```python
from build123d import *

# Parameters (mm, degrees)
SKETCH1_W           = 51
SKETCH1_H           = 36
BOSS_EXTRUDE1_DEPTH = 3
SKETCH2_W           = 45
SKETCH2_H           = 30
BOSS_EXTRUDE2_DEPTH = 10
FILLET1_R           = 1.8
FILLET2_R           = 2.2
CHAMFER1_SIZE       = 1
SKETCH3_R           = 15
CUT_EXTRUDE1_DEPTH  = 10
SKETCH4_R           = 1.25
CUT_EXTRUDE2_DEPTH  = 50
CHAMFER2_SIZE       = 1
SKETCH5_R           = 4.5
BOSS_EXTRUDE3_DEPTH = 7


with BuildPart() as part:
    # Sketch1 → Boss-Extrude1 (new body)
    with BuildSketch(Plane(origin=(0, 0, 0), x_dir=(1, 0, 0), z_dir=(0, 1, 0))):
        Rectangle(SKETCH1_W, SKETCH1_H)
    extrude(amount=BOSS_EXTRUDE1_DEPTH)

    # Sketch2 → Boss-Extrude2 (add)
    with BuildSketch(Plane(origin=(0, 3, 0), x_dir=(1, 0, 0), z_dir=(0, 1, 0))):
        Polygon((-22.5, 18), (-25.5, 18), (-25.5, 15), (-25.5, -15), (-25.5, -18), (-22.5, -18), (22.5, -18), (25.5, -18), (25.5, -15), (25.5, 15), (25.5, 18), (22.5, 18), align=None)
        Rectangle(SKETCH2_W, SKETCH2_H, mode=Mode.SUBTRACT)
    extrude(amount=BOSS_EXTRUDE2_DEPTH)

    # Fillet1
    fillet1_edges = [part.edges().sort_by_distance(p)[0] for p in [
        (22.5, 8, 15),
        (-22.5, 8, 15),
        (-22.5, 8, -15),
        (22.5, 8, -15),
    ]]
    fillet(fillet1_edges, radius=FILLET1_R)

    # Fillet2
    fillet2_edges = [part.edges().sort_by_distance(p)[0] for p in [
        (25.5, 6.5, 18),
        (-25.5, 6.5, 18),
        (-25.5, 6.5, -18),
        (25.5, 6.5, -18),
    ]]
    fillet(fillet2_edges, radius=FILLET2_R)

    # Chamfer1
    chamfer1_edges = [part.edges().sort_by_distance(p)[0] for p in [
        (-25.5, 0, 0),
        (25.5, 0, 0),
        (0, 0, 18),
        (0, 0, -18),
        (24.855634919, 0, 17.355634919),
        (24.855634919, 0, -17.355634919),
        (-24.855634919, 0, 17.355634919),
        (-24.855634919, 0, -17.355634919),
    ]]
    chamfer(chamfer1_edges, length=CHAMFER1_SIZE)

    # Sketch3 → Cut-Extrude1 (cut)
    with BuildSketch(Plane(origin=(0, 3, 0), x_dir=(1, 0, 0), z_dir=(0, 1, 0))):
        with Locations(Location((0, 0, 0), (0, 0, 90))):
            Circle(SKETCH3_R)
    extrude(amount=-CUT_EXTRUDE1_DEPTH, mode=Mode.SUBTRACT)

    # Sketch4 → Cut-Extrude2 (cut)
    with BuildSketch(Plane.XY.offset(18)):
        with Locations((-13.2, 5.8)):
            Circle(SKETCH4_R)
        with Locations((13.2, 5.8)):
            Circle(SKETCH4_R)
    extrude(amount=-CUT_EXTRUDE2_DEPTH, mode=Mode.SUBTRACT)

    # Chamfer2
    chamfer2_edges = [part.edges().sort_by_distance(p)[0] for p in [
        (-25.5, 13, 0),
        (0, 13, -18),
        (0, 13, 18),
        (25.5, 13, 0),
        (24.855634919, 13, 17.355634919),
        (24.855634919, 13, -17.355634919),
        (-24.855634919, 13, 17.355634919),
        (-24.855634919, 13, -17.355634919),
    ]]
    chamfer(chamfer2_edges, length=CHAMFER2_SIZE)

    # Sketch5 → Boss-Extrude3 (add)
    with BuildSketch(Plane(origin=(0, 0, -18), x_dir=(-1, 0, 0), z_dir=(0, 0, -1))):
        with Locations(Location((0, 6.6, 0), (0, 0, 180))):
            Circle(SKETCH5_R)
    extrude(amount=BOSS_EXTRUDE3_DEPTH)


solid = part.part
```
Build history of the part. All positions in model axes, mm. A direction names the side the tool comes from. Round coordinates to 2 decimals unless told otherwise and drop trailing zeros. Write each loop counter-clockwise with the first axis right and the second up, starting at its lowest first coordinate (ties: lowest second). Pieces come first, ordered by that corner, then holes.
1) Mould opens along Y. For faces 3 (the cylindrical face through (-12.045, 5.321, 16.521)), 4 (the flat face through (-25.5, 6, 0)), 5 (the flat face through (-0.3, 0, -15.3)), 6 (the cylindrical face through (14.355, 5.321, -16.479)) say: +Y half, -Y half, draft (parallel to the pull), parting line (faces both ways), or undercut.
2) Band-saw the part on A-A, the plane z = 0. List the corners of the cut face in (x, y).
3) 3-axis set-ups, long thin cutter, end or side, ignore diameter. For faces 1 (the cylindrical face through (-21.987, 8.07, -14.459)), 2 (the flat face through (0, 13, 16)): which of +Z, -Z, +X, -X, +Y, -Y reach the whole face in a straight line?
4) Band-saw the part on D-D, the plane z = 7.5. List the corners of the cut face in (x, y), and give its area (3 significant figures).
5) Drill centre lines: probe 1 along Y at (x, z) = (13.2, 16.05); probe 2 along X at (y, z) = (9, -13); probe 3 along Z at (x, y) = (6.5, 3.75). Where is each one in solid material? Low to high.
6) Band-saw the part on B-B, the plane x = -16. List the corners of the cut face in (y, z), and give its area (3 significant figures).
7) Pin check, flat tips, straight feed: pin 1 (18 mm diameter, centred on x = 6, z = -7.5, fed in from +Y); pin 2 (4 mm diameter, centred on x = 13.2, y = 5.8, fed in from -Z); pin 3 (2 mm diameter, centred on x = -13.2, y = 5.8, fed in from +Z). Stop position of each tip, or through.
8) Band-saw the part on C-C, the plane y = 8.5. List the corners of the cut face in (x, z).
Ans:
1. face 3: undercut
1. face 4: draft
1. face 5: -Y half
1. face 6: undercut
2. outline: (-25.5, 1) - (-24.5, 0) - (-15, 0) - (-15, 3) - (-22.5, 3) - (-22.5, 13) - (-24.5, 13) - (-25.5, 12) - close; (15, 0) - (24.5, 0) - (25.5, 1) - (25.5, 12) - (24.5, 13) - (22.5, 13) - (22.5, 3) - (15, 3) - close
3. face 1: +Y
3. face 2: +Z, -Z, +X, -X, +Y
4. outline: (-25.5, 1) - (-24.5, 0) - (-12.99, 0) - (-12.99, 3) - (-22.5, 3) - (-22.5, 13) - (-24.5, 13) - (-25.5, 12) - close; (12.99, 0) - (24.5, 0) - (25.5, 1) - (25.5, 12) - (24.5, 13) - (22.5, 13) - (22.5, 3) - (12.99, 3) - close
4. area: 133 mm2
5. probe 1: y = 0 to 4.55, 7.05 to 13
5. probe 2: x = -25.5 to -22.5, 22.5 to 25.5
5. probe 3: z = -18 to -15, 15 to 18
6. outline: (0, -17) - (1, -18) - (12, -18) - (13, -17) - (13, -15) - (3, -15) - (3, 15) - (13, 15) - (13, 17) - (12, 18) - (1, 18) - (0, 17) - close
6. area: 166 mm2
7. pin 1: stops at y = 13
7. pin 2: stops at z = -18
7. pin 3: passes through
8. outline: (-25.5, -15.8) arc R2.2 ccw to (-23.3, -18) - (-4.08, -18) - (-4.08, -25) - (4.08, -25) - (4.08, -18) - (23.3, -18) arc R2.2 ccw to (25.5, -15.8) - (25.5, 15.8) arc R2.2 ccw to (23.3, 18) - (-23.3, 18) arc R2.2 ccw to (-25.5, 15.8) - close; hole (-22.5, -13.2) arc R1.8 ccw to (-20.7, -15) - (20.7, -15) arc R1.8 ccw to (22.5, -13.2) - (22.5, 13.2) arc R1.8 ccw to (20.7, 15) - (-20.7, 15) arc R1.8 ccw to (-22.5, 13.2) - close
